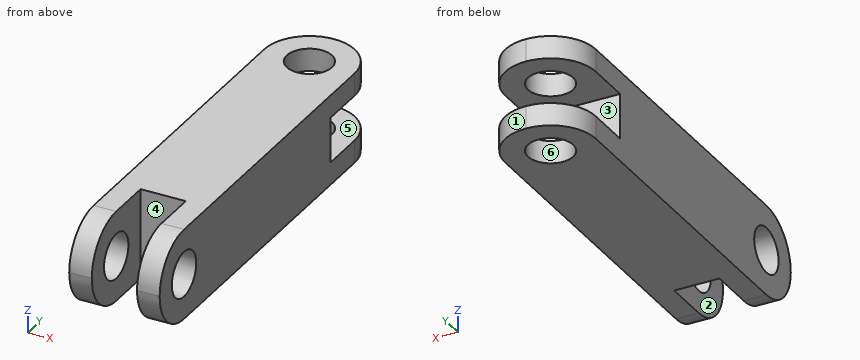
from build123d import *

# Parameters (mm, degrees)
SKETCH2_W               = 101.6
SKETCH2_H               = 101.6
BOSS_EXTRUDE1_DEPTH     = 457.2
CUT_EXTRUDE1_DEPTH      = 463.810025821
CUT_EXTRUDE1_DEPTH_BACK = 463.810025821
SKETCH3_R               = 25.4
SKETCH3_W               = 50.8
SKETCH3_H               = 101.6
FILLET1_R               = 50.8
CUT_EXTRUDE2_DEPTH      = 472.099819571
CUT_EXTRUDE2_DEPTH_BACK = 472.099819571
SKETCH4_R               = 25.4
SKETCH4_W               = 50.8
SKETCH4_H               = 101.6


with BuildPart() as part:
    # Sketch2 → Boss-Extrude1 (new body)
    with BuildSketch(Plane(origin=(0, 0, 0), x_dir=(1, 0, 0), z_dir=(0, 1, 0))):
        Rectangle(SKETCH2_W, SKETCH2_H)
    extrude(amount=BOSS_EXTRUDE1_DEPTH)

    # Sketch3 → Cut-Extrude1 (cut, two sides: drawn at the far end of the back side and taken through both)
    with BuildSketch(Plane.XY.offset(-CUT_EXTRUDE1_DEPTH_BACK)):
        with Locations((0, 406.4)):
            Circle(SKETCH3_R)
        with Locations((0, 50.8)):
            Rectangle(SKETCH3_W, SKETCH3_H)
    extrude(amount=CUT_EXTRUDE1_DEPTH + CUT_EXTRUDE1_DEPTH_BACK, mode=Mode.SUBTRACT)

    # Fillet1
    fillet1_edges = [part.edges().sort_by_distance(p)[0] for p in [
        (-38.1, 0, -50.8),
        (-38.1, 0, 50.8),
        (38.1, 0, -50.8),
        (38.1, 0, 50.8),
        (-50.8, 457.2, 0),
        (50.8, 457.2, 0),
    ]]
    fillet(fillet1_edges, radius=FILLET1_R - 0.0001)  # a hair under: the kernel refuses the full size

    # Sketch4 → Cut-Extrude2 (cut, two sides: drawn at the far end of the back side and taken through both)
    with BuildSketch(Plane(origin=(50.8, 0, 0), x_dir=(0, 0, -1), z_dir=(1, 0, 0)).offset(-CUT_EXTRUDE2_DEPTH_BACK)):
        with Locations((0, 50.8)):
            Circle(SKETCH4_R)
        with Locations((0, 406.4)):
            Rectangle(SKETCH4_W, SKETCH4_H)
    extrude(amount=CUT_EXTRUDE2_DEPTH + CUT_EXTRUDE2_DEPTH_BACK, mode=Mode.SUBTRACT)


solid = part.part
Geometry: final body of the model. Coordinates: model frame, mm. Face numbers are marked on the shaded views. A direction names the side the tool comes from. Give positions to 0.01 mm unless a question says otherwise; leave off trailing zeros. Write each loop counter-clockwise with the first axis right and the second up, starting at its lowest first coordinate (ties: lowest second). Pieces come first, ordered by that corner, then holes. Notation, with made-up numbers: (54.25, 49.5) -> (92.25, 49.5) arc R38 ccw to (92.25, 87.5) -> close; hole circle Ø2 at (-31, -35). An arc over 180 degrees is marked (long way). Answer as a JSON object with one key per item and string values.
1. Access query for the marked faces 4, 5 and 6. Directions: +Z, -Z, +X, -X, +Y, -Y. A direction counts if a zero-diameter tool reaches every point of the face in a straight line with its end or side. Return the directions, or none.
Ans:
{"face 4": "+Z, -Z, -Y", "face 5": "+X, -X, +Y", "face 6": "+Z, -Z"}
2. Cut plane A-A on y = 31.5. Output: boundary loops of the cut face in (x, z).
Ans:
{"outline": "(-50.8, -46.99) -> (-25.4, -46.99) -> (-25.4, -16.51) -> (-50.8, -16.51) -> close; (-50.8, 16.51) -> (-25.4, 16.51) -> (-25.4, 46.99) -> (-50.8, 46.99) -> close; (25.4, -46.99) -> (50.8, -46.99) -> (50.8, -16.51) -> (25.4, -16.51) -> close; (25.4, 16.51) -> (50.8, 16.51) -> (50.8, 46.99) -> (25.4, 46.99) -> close"}
3. Contact query for flat-ended pins moving along their axis: pin 1 (3 mm diameter, centred on x = 14.5, z = -13.5, fed in from +Y); pin 2 (1.5 mm diameter, centred on x = 40.5, z = -25, fed in from +Y); pin 3 (6 mm diameter, centred on x = 8.5, z = -33, fed in from +Y). Output: stop coordinate, or through.
Ans:
{"pin 1": "stops at y = 355.6", "pin 2": "stops at y = 437.89", "pin 3": "stops at y = 456.9"}
4. Cut plane B-B on z = 20. Output: boundary loops of the cut face in (x, y), and give its area (3 significant figures).
Ans:
{"outline": "(-50.8, 4.1) -> (-25.4, 4.1) -> (-25.4, 35.14) -> (-50.8, 35.14) -> close; (-50.8, 66.46) -> (-25.4, 66.46) -> (-25.4, 101.6) -> (25.4, 101.6) -> (25.4, 66.46) -> (50.8, 66.46) -> (50.8, 355.6) -> (-50.8, 355.6) -> close; (25.4, 4.1) -> (50.8, 4.1) -> (50.8, 35.14) -> (25.4, 35.14) -> close", "area": "29,200 mm^2"}
5. Mould query, pull axis X, two halves, no side actions, for the marked faces 1, 2 and 3. Classes: pulls with the +X half, pulls with the -X half, needs draft (parallel to the pull), parting line crosses it, or undercut.
Ans:
{"face 1": "pulls with the +X half", "face 2": "undercut", "face 3": "needs draft"}
6. Ray query, probe 1 along X at (y, z) = (76.5, 34.5); probe 2 along Z at (x, y) = (44, 50); probe 3 along Y at (x, z) = (-36, 0). Return the intervals inside material, ascending. Write a range as from..to.
Ans:
{"probe 1": "x = -50.8..-25.4, 25.4..50.8", "probe 2": "z = -50.79..-25.39, 25.39..50.79", "probe 3": "y = 0..25.4, 76.2..355.6"}
